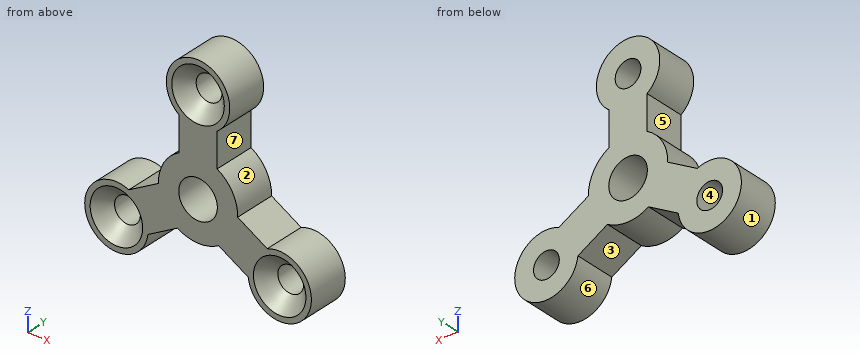
from build123d import *

# Parameters (mm, degrees)
F0_R     = 3.175
F0_R_2   = 4.7625
F1_DEPTH = 10.16
F2_SIZE  = 3.302


with BuildPart() as f1:
    # F0 (on Front) → F1 (new body)
    with BuildSketch(Plane.XZ):
        with BuildLine():
            Line((4.699, 8.576027), (4.699, 16.986253))
            ThreePointArc((4.699, 16.986253), (0, 31.0642), (-4.699, 16.986253))
            Line((-4.699, 16.986253), (-4.699, 8.576027))
            ThreePointArc((-4.699, 8.576027), (-8.468862, 4.8895), (-9.776557, -0.21856))
            Line((-9.776557, -0.21856), (-17.060027, -4.423673))
            ThreePointArc((-17.060027, -4.423673), (-26.902386, -15.5321), (-12.361027, -12.56258))
            Line((-12.361027, -12.56258), (-5.077557, -8.357467))
            ThreePointArc((-5.077557, -8.357467), (0, -9.779), (5.077557, -8.357467))
            Line((5.077557, -8.357467), (12.361027, -12.56258))
            ThreePointArc((12.361027, -12.56258), (26.902386, -15.5321), (17.060027, -4.423673))
            Line((17.060027, -4.423673), (9.776557, -0.21856))
            ThreePointArc((9.776557, -0.21856), (8.468862, 4.8895), (4.699, 8.576027))
        make_face()
        with Locations((-20.127296, -11.6205)):
            Circle(F0_R, mode=Mode.SUBTRACT)
        Circle(F0_R_2, mode=Mode.SUBTRACT)
        with Locations((20.127296, -11.6205)):
            Circle(F0_R, mode=Mode.SUBTRACT)
        with Locations((0, 23.241)):
            Circle(F0_R, mode=Mode.SUBTRACT)
    extrude(amount=-F1_DEPTH)

    # F2
    f2_edges = [f1.edges().sort_by_distance(p)[0] for p in [
        (-3.175, 0, 23.241),
        (-23.302296, 0, -11.6205),
        (16.952296, 0, -11.6205),
    ]]
    chamfer(f2_edges, length=F2_SIZE)


solid = f1.part
The model under review builds one solid part; all positions refer to its coordinate system, in mm. Face numbers are marked on the shaded views. A direction names the side the tool comes from. Give positions to 0.01 mm unless a question says otherwise; leave off trailing zeros. Order: outer loops, then holes, each group sorted by start corner. A loop starts at its lowest first (then second) coordinate and runs counter-clockwise, first axis right, second up. Notation, with made-up numbers: M 88,-32.5 L 128,-32.5 A8 ccw 128,-27.5 Z; hole C 74,-24.75 d8. An arc over 180 degrees is marked long. Answer in a Markdown table with one row per item. Add a question column.
1. Add section B-B on z = -2. State the section outline as (x, y) points.
2. Add section C-C on y = 5.75. Count the separate pieces of the cut face and the enclosed holes in it, plus the area to 3 significant figures.
3. Add section A-A on x = 0. State the section outline as (y, z) points.
4. For pin 1 Ø2.5 at (y, z) = (2.5, 11) entering from +X; pin 2 Ø8.5 at (x, z) = (-20.13, -11.62) entering from -Y; pin 3 Ø5 at (y, z) = (8, 15.5) entering from +X; pin 4 Ø5 at (x, z) = (0, 23.241) entering from -Y, all flat-tipped, find the tip position at first contact; note any pin that passes through.
5. To check wall thickness, follow line 1 along Z through (x, y) = (0, 7.25); line 2 along X through (y, z) = (7, -14); line 3 along X through (y, z) = (8, -13.5). State the ranges of each line that lie inside material, in increasing order.
6. Mouldability with a two-part tool opening along X and no side actions: class the marked faces 4, 5, 6 and 7 as released by +X, released by -X, zero draft, split by the parting line, or undercut.
7. Machinability: for the marked faces 1, 2 and 3, which of the approach directions +Z, -Z, +X, -X, +Y, -Y give a long, thin tool a straight path to every point of the face, cutting with its end or side? Answer none if there is none.
The answers:
| question | item | result |
|---|---|---|
| 1 | outline | M -12.86,0 L -4.32,0 L -4.32,10.16 L -12.86,10.16 Z; M 4.32,0 L 12.86,0 L 12.86,10.16 L 4.32,10.16 Z |
| 2 | separate pieces | 1 |
| 2 | enclosed holes | 4 |
| 2 | area | 895 mm2 |
| 3 | outline | M 0,-9.78 L 10.16,-9.78 L 10.16,-4.76 L 0,-4.76 Z; M 0,4.76 L 10.16,4.76 L 10.16,20.07 L 3.3,20.07 L 0,16.76 Z; M 0,29.72 L 3.3,26.42 L 10.16,26.42 L 10.16,31.06 L 0,31.06 Z |
| 4 | pin 1 | x = 4.7 |
| 4 | pin 2 | y = 2.22 |
| 4 | pin 3 | x = 5.81 |
| 4 | pin 4 | through |
| 5 | line 1 | -9.78 to -4.76, 4.76 to 20.07, 26.42 to 31.06 |
| 5 | line 2 | -27.58 to -22.23, -18.03 to -12.67, 12.67 to 18.03, 22.23 to 27.58 |
| 5 | line 3 | -27.72 to -22.69, -17.57 to -12.53, 12.53 to 17.57, 22.69 to 27.72 |
| 6 | face 4 | undercut |
| 6 | face 5 | released by -X |
| 6 | face 6 | undercut |
| 6 | face 7 | released by +X |
| 7 | face 1 | +Y, -Y |
| 7 | face 2 | +X, +Y, -Y |
| 7 | face 3 | -Z, +Y, -Y |
